The listing builds one solid part. Answer for the finished solid, in the listing's coordinates (mm). A direction names the side the tool comes from. Round coordinates to 2 decimals unless told otherwise and drop trailing zeros. Order: outer loops, then holes, each group sorted by start corner. A loop starts at its lowest first (then second) coordinate and runs counter-clockwise, first axis right, second up. Notation, with made-up numbers: (24, -5) - (40, -5) arc R26 cw to (40, 23) - close; hole circle Ø5 at (-33.5, 46). An arc over 180 degrees is marked (long way). Use CSV: the item, a comma, the result in double quotes. Start each with the question number.
Item 1: Find section B-B, the plane y = 14. Give the vertices of the cut face in (x, z).
Item 2: Flat-ended cylindrical pins translate along their axes: P1, Ø3, axis at x = -5, y = 0.5, coming from the -Z side; P2, Ø1, axis at x = -6, y = 11.5, coming from the +Z side; P3, Ø2, axis at x = 4, z = 3.5, coming from the +Y side; P4, Ø3.5, axis at y = 11, z = 2, coming from the +X side. Find the tip coordinate at first contact, or state that the pin passes through.
Item 3: Determine the mould class of faces 1 (the flat face through (-9, 7, 3)), 2 (the flat face through (-6, 14, 2.43)), 3 (the flat face through (-4.757, -25.444, 3.295)) for opening direction X: +X half, -X half, draft (parallel to the pull), parting line (faces both ways), or undercut.
Item 4: Find section C-C, the plane x = -6.75. Give the vertices of the cut face in (y, z).
Item 5: Find section A-A, the plane z = 3.25. Give the vertices of the cut face in (x, y), plus the area to 3 significant figures.
Item 6: Find section D-D, the plane y = -7. Give the vertices of the cut face in (x, z).
Item 7: For faces 4 (the cylindrical face through (-11.5, 13.6, 3.2)), 5 (the flat face through (-5.25, -1, 3)), 6 (the flat face through (-6, 14, 4.07)), 7 (the flat face through (4, -3, 3)), determine the directions among +Z, -Z, +X, -X, +Y, -Y from which every point of the face is accessible in a straight line to the end or side of a thin tool.
Item 8: Straight lines are drawn through the part: line 1 along X through (y, z) = (-17, 5.75); line 2 along Y through (x, z) = (-10.25, 4.5); line 3 along X through (y, z) = (-1, 6.25). For each, find the intervals that lie inside material, in ascending order. Write a range as [from, to].
```python
from build123d import *

# Parameters (mm, degrees)
SZKIC1_W                    = 10.5
SZKIC1_H                    = 40
DODANIE_WYCI_GNI_CIE1_DEPTH = 6.5
SZKIC2_W                    = 2.5
SZKIC2_H                    = 8
WYTNIJ_WYCI_GNI_CIE1_DEPTH  = 6.5
SFAZOWANIE1_SIZE            = 0.5
DODANIE_WYCI_GNI_CIE2_DEPTH = 13
SZKIC4_W                    = 10.5
SZKIC4_H                    = 9.5
DODANIE_WYCI_GNI_CIE3_DEPTH = 6.5
SFAZOWANIE2_SIZE            = 8
SFAZOWANIE2_SIZE2           = 1
SFAZOWANIE3_SIZE            = 1
SFAZOWANIE3_SIZE2           = 8
SFAZOWANIE4_SIZE            = 2


with BuildPart() as part:
    # Szkic1 → Dodanie-wyciągnięcie1 (new body)
    with BuildSketch(Plane.XY):
        Rectangle(SZKIC1_W, SZKIC1_H)
    extrude(amount=DODANIE_WYCI_GNI_CIE1_DEPTH)

    # Szkic2 → Wytnij-wyciągnięcie1 (cut)
    with BuildSketch(Plane.XY.offset(6.5)):
        with Locations((4, 1)):
            Rectangle(SZKIC2_W, SZKIC2_H)
        Polygon((5.25, 20), (-0.25, 20), (-0.25, 5), (2.75, 5), (5.25, 5), align=None)
    extrude(amount=-WYTNIJ_WYCI_GNI_CIE1_DEPTH, mode=Mode.SUBTRACT)

    # Sfazowanie1
    sfazowanie1_edges = [part.edges().sort_by_distance(p)[0] for p in [
        (1.25, 5, 0),
        (2.75, 5, 3.25),
        (1.25, 5, 6.5),
    ]]
    chamfer(sfazowanie1_edges, length=SFAZOWANIE1_SIZE)

    # Szkic3 → Dodanie-wyciągnięcie2 (add)
    with BuildSketch(Plane(origin=(0, 20, 0), x_dir=(1, 0, 0), z_dir=(0, 1, 0))):
        with BuildLine():
            ThreePointArc((-7.258694583, -2.429590228), (-11.5, -3.25), (-7.258694583, -4.070409772))
            Line((-7.258694583, -4.070409772), (-9.3, -4.070409772))
            Line((-9.3, -4.070409772), (-9.3, -2.429590228))
            Line((-9.3, -2.429590228), (-7.258694583, -2.429590228))
        make_face()
        with BuildLine():
            Line((-9.3, -4.070409772), (-7.258694583, -4.070409772))
            ThreePointArc((-7.258694583, -4.070409772), (-7.140037973, -3.667808618), (-7.1, -3.25))
            ThreePointArc((-7.1, -3.25), (-7.140037973, -2.832191382), (-7.258694583, -2.429590228))
            Line((-7.258694583, -2.429590228), (-9.3, -2.429590228))
            Line((-9.3, -2.429590228), (-9.3, -4.070409772))
        make_face()
        with BuildLine():
            Line((-7.258694583, -4.070409772), (-5.25, -4.070409772))
            Line((-5.25, -4.070409772), (-5.25, -2.429590228))
            Line((-5.25, -2.429590228), (-7.258694583, -2.429590228))
            ThreePointArc((-7.258694583, -2.429590228), (-7.140037973, -2.832191382), (-7.1, -3.25))
            ThreePointArc((-7.1, -3.25), (-7.140037973, -3.667808618), (-7.258694583, -4.070409772))
        make_face()
    extrude(amount=-DODANIE_WYCI_GNI_CIE2_DEPTH)

    # Szkic4 → Dodanie-wyciągnięcie3 (add)
    with BuildSketch(Plane.XY.offset(6.5)):
        with Locations((0, -24.75)):
            Rectangle(SZKIC4_W, SZKIC4_H)
    extrude(amount=-DODANIE_WYCI_GNI_CIE3_DEPTH)

    # Sfazowanie2
    sfazowanie2_edges = [part.edges().sort_by_distance(p)[0] for p in [
        (5.25, -29.5, 3.25),
    ]]
    sfazowanie2_side = [part.faces().sort_by_distance(p)[0] for p in [
        (5.25, -16.25, 3.25),
    ]]
    chamfer(sfazowanie2_edges, length=SFAZOWANIE2_SIZE, length2=SFAZOWANIE2_SIZE2, reference=sfazowanie2_side[0])

    # Sfazowanie3
    sfazowanie3_edges = [part.edges().sort_by_distance(p)[0] for p in [
        (-5.25, -29.5, 3.25),
    ]]
    sfazowanie3_side = [part.faces().sort_by_distance(p)[0] for p in [
        (-0.5, -29.5, 3.25),
    ]]
    chamfer(sfazowanie3_edges, length=SFAZOWANIE3_SIZE, length2=SFAZOWANIE3_SIZE2, reference=sfazowanie3_side[0])

    # Sfazowanie4
    sfazowanie4_edges = [part.edges().sort_by_distance(p)[0] for p in [
        (0, -29.5, 0),
    ]]
    chamfer(sfazowanie4_edges, length=SFAZOWANIE4_SIZE)


solid = part.part
```
Worked out:
1,outline,"(-7.26, 2.43) - (-5.25, 2.43) - (-5.25, 0) - (-0.25, 0) - (-0.25, 6.5) - (-5.25, 6.5) - (-5.25, 4.07) - (-7.26, 4.07) arc R2.2 ccw (long way) to start"
2,P1,"stops at z = 0"
2,P2,"stops at z = 4.07"
2,P3,"stops at y = -3"
2,P4,"stops at x = -0.25"
3,face 1,"draft"
3,face 2,"undercut"
3,face 3,"-X half"
4,outline,"(7, 2.43) - (20, 2.43) - (20, 4.07) - (7, 4.07) - close"
5,outline,"(-11.5, 7) - (-5.25, 7) - (-5.25, -21.5) - (-4.25, -29.5) - (4.25, -29.5) - (5.25, -21.5) - (5.25, -3) - (2.75, -3) - (2.75, 4.5) - (2.25, 5) - (-0.25, 5) - (-0.25, 20) - (-11.5, 20) - close"
5,area,"490 mm²"
6,outline,"(-5.25, 0) - (5.25, 0) - (5.25, 6.5) - (-5.25, 6.5) - close"
7,face 4,"+Y, -Y"
7,face 5,"-Y"
7,face 6,"+Z, +Y, -Y"
7,face 7,"+Z, -Z, +X, +Y"
8,line 1,"x = [-5.25, 5.25]"
8,line 2,"y = [7, 20]"
8,line 3,"x = [-5.25, 2.75]"
